```python
from build123d import *

# Parameters (mm, degrees)
F1_DEPTH = 17
F3_DEPTH = 2
F4_R     = 1.99999


# Not quite as in the source:
# - a fillet or chamfer is up to 0.001 mm smaller than in the source, because OpenCascade refuses the exact size
# - a feature of the source that left no trace in its solid (it failed there, or was rolled back) is left out


with BuildPart() as f1:
    # F0 (on Right) → F1 (new body)
    with BuildSketch(Plane.YZ):
        with BuildLine():
            Line((-1.8, 0), (0, 0))
            Line((0, 0), (0, 40))
            ThreePointArc((0, 40), (8.5, 48.5), (17, 40))
            Line((17, 40), (17, 0))
            Line((17, 0), (18.8, 0))
            Line((18.8, 0), (18.8, 40))
            ThreePointArc((18.8, 40), (8.5, 50.3), (-1.8, 40))
            Line((-1.8, 40), (-1.8, 0))
        make_face()
    extrude(amount=F1_DEPTH)

    # F2 (on face) → F3 (join)
    with BuildSketch(Plane.YZ.offset(17)):
        with BuildLine():
            ThreePointArc((-1.8, 40), (8.5, 50.3), (18.8, 40))
            Line((18.8, 40), (18.8, 0))
            Line((18.8, 0), (23.8, 0))
            Line((23.8, 0), (23.8, 40))
            ThreePointArc((23.8, 40), (8.5, 55.3), (-6.8, 40))
            Line((-6.8, 40), (-6.8, 0))
            Line((-6.8, 0), (-1.8, 0))
            Line((-1.8, 0), (-1.8, 40))
        make_face()
        with BuildLine():
            Line((18.8, 0), (18.8, 40))
            ThreePointArc((18.8, 40), (8.5, 50.3), (-1.8, 40))
            Line((-1.8, 40), (-1.8, 0))
            Line((-1.8, 0), (0, 0))
            Line((0, 0), (0, 40))
            ThreePointArc((0, 40), (8.5, 48.5), (17, 40))
            Line((17, 40), (17, 0))
            Line((17, 0), (18.8, 0))
        make_face()
    extrude(amount=F3_DEPTH)

    # F4 (radius 2 in the source; OpenCascade refuses exactly that, so slightly less here)
    f4_edges = [f1.edges().sort_by_distance(p)[0] for p in [
        (19, -6.8, 20),
        (19, 8.5, 55.3),
        (19, 23.8, 20),
    ]]
    fillet(f4_edges, radius=F4_R)


solid = f1.part
```
Here's how the part is built. I have some questions about the finished solid (model axes, mm). A direction names the side the tool comes from. Coordinates: 2 decimals unless noted, no trailing zeros. Write each loop counter-clockwise with the first axis right and the second up, starting at its lowest first coordinate (ties: lowest second). Pieces come first, ordered by that corner, then holes. Notation, with made-up numbers: (-24, -25.75) -> (-8, -25.75) arc R9 cw to (-8, -12.75) -> close; hole circle Ø2 at (-28.5, 52). An arc over 180 degrees is marked (long way). Use a Markdown table: item, result. Add a question column.
(1) For faces 1 (the flat face through (8, 18.8, 20)), 2 (the flat face through (8, -1.8, 20)), 3 (the flat face through (9, 17, 20)), which set-ups out of +Z, -Z, +X, -X, +Y, -Y let a thin tool reach every point of the face, with its end or its side?
(2) We'd pull the mould along Y, two halves only. Please class faces 4 (the cylindrical face through (8.4, 8.7, 50.3)), 5 (the flat face through (17, -2, 28)), 6 (the cylindrical face through (9.367, 8.313, 48.498)): +Y half, -Y half, draft (parallel to the pull), parting line (faces both ways), or undercut.
(3) Please list where these lines run through material, in increasing order: line 1 (Y direction, x = 4, z = 39); line 2 (Y direction, x = 10, z = 46); line 3 (X direction, y = -3, z = 36.5).
(4) I'm going to push flat-ended pins straight in: P1, Ø4, axis at x = 5.5, z = 35, coming from the -Y side; P2, Ø3, axis at x = 7, y = 6.5, coming from the -Z side; P3, Ø2, axis at y = 4, z = 43.5, coming from the +X side; P4, Ø10, axis at x = 15, y = 14, coming from the +Z side. Where does each tip first touch, or does it pass through?
(5) If we section it at B-B, the plane x = 11.25: Write out the boundary of the cut face in (y, z), and give its area (3 significant figures).
Outcome:
| question | item | result |
|---|---|---|
| 1 | face 1 | +Z, -Z, -X, +Y |
| 1 | face 2 | +Z, -Z, -X, -Y |
| 1 | face 3 | -Z, +X, -X |
| 2 | face 4 | parting line |
| 2 | face 5 | draft |
| 2 | face 6 | undercut |
| 3 | line 1 | y = -1.8 to 0, 17 to 18.8 |
| 3 | line 2 | y = 0.13 to 2.48, 14.52 to 16.87 |
| 3 | line 3 | x = 17 to 19 |
| 4 | P1 | stops at y = -1.8 |
| 4 | P2 | stops at z = 47.75 |
| 4 | P3 | passes through |
| 4 | P4 | stops at z = 55.27 |
| 5 | outline | (-1.8, 0) -> (0, 0) -> (0, 40) arc R8.5 cw to (17, 40) -> (17, 0) -> (18.8, 0) -> (18.8, 40) arc R10.3 ccw to (-1.8, 40) -> close |
| 5 | area | 197 mm^2 |
